Check sheet for the modelled part. Datum: model origin and axes. Units: mm. A direction names the side the tool comes from. Give positions to 0.01 mm unless a question says otherwise; leave off trailing zeros. Loops run counter-clockwise (first coordinate to the right, second up) from the corner with the lowest first, then second, coordinate; pieces in that order, holes last. Notation, with made-up numbers: (49.5, 7.25) - (75.5, 7.25) arc R21 ccw to (75.5, 42.25) - close; hole circle Ø1 at (33.5, -17). An arc over 180 degrees is marked (long way). Answer in a Markdown table with one row per item. Add a question column.
(1) Sectioned sample at A-A on z = 4. Enter the section's corners in (x, y).
(2) Sectioned sample at C-C on x = -27. Enter the section's corners in (y, z).
(3) Sectioned sample at D-D on x = 16. Enter the section's corners in (y, z), then the cut area to 3 significant figures.
(4) Go/stop test with flat-tipped pins: P1, Ø1.5, axis at x = 17.5, y = -4.5, coming from the +Z side; P2, Ø1.2, axis at x = 3, z = 1.5, coming from the -Y side; P3, Ø1, axis at x = -4.5, z = 3.5, coming from the +Y side; P4, Ø1.2, axis at y = 1.5, z = 2, coming from the -X side. Record where each tip stops, or that it passes through.
(5) Sectioned sample at B-B on y = -13. Enter the section's corners in (x, z), then the cut area to 3 significant figures.
(6) Thickness scan on L1, parallel to Y at x = -27, z = 5.45; L2, parallel to Y at x = 27, z = 2.9; L3, parallel to Y at x = 0, z = 0.5. Record the ranges inside material, lowest first.
(7) Draft check along Y on faces 1 (the face through (0, 0, 0)), 2 (the face through (-29.43, 8.17, 1.23)), 3 (the face through (-21.43, -8.616, 1.232)), 4 (the face through (24.636, -11.234, 1.232)). Enter one of: released by +Y, released by -Y, zero draft, split by the parting line, or undercut.
(8) Set-up check for faces 5 (the face through (-25, 14, 4.8)), 6 (the face through (-22, 7.57, 1)), 7 (the face through (4, 14.05, 1)): record each of +Z, -Z, +X, -X, +Y, -Y from which the full face is reachable in a straight line by a thin tool's end or side.
from build123d import *

# Parameters (mm, degrees)
SKETCH003_R   = 1.6
PAD_DEPTH     = 2.5
SKETCH_R      = 3
SKETCH_R_2    = 1.6
PAD001_DEPTH  = 2.3
SKETCH004_R   = 3
SKETCH004_R_2 = 2.5
PAD002_DEPTH  = 2
SKETCH005_W   = 26.6
SKETCH005_H   = 19.6
POCKET_DEPTH  = 1.5


with BuildPart() as part:
    # Sketch003 → Pad (new body)
    with BuildSketch(Plane.XY):
        with BuildLine():
            ThreePointArc((-28.087018, -11.203861), (-29.796139, -15.087018), (-25.912982, -16.796139))
            Line((-25.912982, -16.796139), (-0.93534, -7.085908))
            ThreePointArc((-0.210661, -6.95), (-0.579317, -6.984271), (-0.93534, -7.085908))
            Line((9.827812, -6.95), (-0.210661, -6.95))
            ThreePointArc((11.802562, -8.6332), (11.125194, -7.427896), (9.827812, -6.95))
            ThreePointArc((11.802562, -8.6332), (15.79003, -15.309423), (23.276895, -17.411493))
            Line((23.276895, -17.411493), (27.316256, -16.983284))
            ThreePointArc((27.316256, -16.983284), (29.983284, -13.683744), (26.683744, -11.016716))
            Line((22.644383, -11.444926), (26.683744, -11.016716))
            ThreePointArc((17.67, -6.97), (19.160409, -10.315499), (22.644383, -11.444926))
            Line((17.67, 14.05), (17.67, -6.97))
            Line((17.67, 14.05), (-10.570113, 14.05))
            ThreePointArc((-10.570113, 14.05), (-11.282503, 13.751783), (-11.57, 13.035))
            ThreePointArc((-12.569887, 12.02), (-11.857497, 12.318217), (-11.57, 13.035))
            Line((-23, 12.02), (-12.569887, 12.02))
            ThreePointArc((-24, 13.02), (-23.707107, 12.312893), (-23, 12.02))
            Line((-24, 13.02), (-24, 14))
            ThreePointArc((-24, 14), (-27, 17), (-30, 14))
            Line((-30, 14), (-30, 9.57))
            ThreePointArc((-30, 9.57), (-29.414214, 8.155786), (-28, 7.57))
            Line((-17.12, 7.57), (-28, 7.57))
            ThreePointArc((-14.583624, -5.954324), (-10.239947, 1.860298), (-17.12, 7.57))
            Line((-28.087018, -11.203861), (-14.583624, -5.954324))
        make_face()
        with Locations((-27, 14)):
            Circle(SKETCH003_R, mode=Mode.SUBTRACT)
        with Locations((27, -14)):
            Circle(SKETCH003_R, mode=Mode.SUBTRACT)
        with Locations((-27, -14)):
            Circle(SKETCH003_R, mode=Mode.SUBTRACT)
    extrude(amount=PAD_DEPTH)

    # Sketch → Pad001 (new body)
    with BuildSketch(Plane.XY.offset(2.5)):
        with Locations((-27, 14)):
            Circle(SKETCH_R)
        with Locations((-27, 14)):
            Circle(SKETCH_R_2, mode=Mode.SUBTRACT)
        with Locations((27, -14)):
            Circle(SKETCH_R)
        with Locations((27, -14)):
            Circle(SKETCH_R_2, mode=Mode.SUBTRACT)
        with Locations((-27, -14)):
            Circle(SKETCH_R)
        with Locations((-27, -14)):
            Circle(SKETCH_R_2, mode=Mode.SUBTRACT)
    extrude(amount=PAD001_DEPTH)

    # Sketch004 → Pad002 (new body)
    with BuildSketch(Plane.XY.offset(4.8)):
        with Locations((-27, 14)):
            Circle(SKETCH004_R)
        with Locations((-27, 14)):
            Circle(SKETCH004_R_2, mode=Mode.SUBTRACT)
        with Locations((-27, -14)):
            Circle(SKETCH004_R)
        with Locations((-27, -14)):
            Circle(SKETCH004_R_2, mode=Mode.SUBTRACT)
        with Locations((27, -14)):
            Circle(SKETCH004_R)
        with Locations((27, -14)):
            Circle(SKETCH004_R_2, mode=Mode.SUBTRACT)
    extrude(amount=PAD002_DEPTH)

    # Sketch005 → Pocket (cut)
    with BuildSketch(Plane.XY.offset(2.5)):
        with Locations((3.67, 3.55)):
            Rectangle(SKETCH005_W, SKETCH005_H)
    extrude(amount=-POCKET_DEPTH, mode=Mode.SUBTRACT)


solid = part.part
Reply:
| question | item | result |
|---|---|---|
| 1 | outline | circle Ø6 at (-27, -14); circle Ø6 at (-27, 14); circle Ø6 at (27, -14); hole circle Ø3.2 at (-27, -14); hole circle Ø3.2 at (-27, 14); hole circle Ø3.2 at (27, -14) |
| 2 | outline | (-17, 0) - (-15.6, 0) - (-15.6, 4.8) - (-16.5, 4.8) - (-16.5, 6.8) - (-17, 6.8) - close; (-12.4, 0) - (-10.78, 0) - (-10.78, 2.5) - (-11, 2.5) - (-11, 6.8) - (-11.5, 6.8) - (-11.5, 4.8) - (-12.4, 4.8) - close; (7.57, 0) - (12.4, 0) - (12.4, 4.8) - (11.5, 4.8) - (11.5, 6.8) - (11, 6.8) - (11, 2.5) - (7.57, 2.5) - close; (15.6, 0) - (17, 0) - (17, 6.8) - (16.5, 6.8) - (16.5, 4.8) - (15.6, 4.8) - close |
| 3 | outline | (-15.47, 0) - (14.05, 0) - (14.05, 2.5) - (13.35, 2.5) - (13.35, 1) - (-6.25, 1) - (-6.25, 2.5) - (-15.47, 2.5) - close |
| 3 | area | 44.4 mm^2 |
| 4 | P1 | z = 2.5 |
| 4 | P2 | y = -6.95 |
| 4 | P3 | through |
| 4 | P4 | x = -10.29 |
| 5 | outline | (-29.83, 0) - (-28.25, 0) - (-28.25, 4.8) - (-29.29, 4.8) - (-29.29, 6.8) - (-29.83, 6.8) - close; (-25.75, 0) - (-16.15, 0) - (-16.15, 2.5) - (-24.17, 2.5) - (-24.17, 6.8) - (-24.71, 6.8) - (-24.71, 4.8) - (-25.75, 4.8) - close; (13.57, 0) - (25.75, 0) - (25.75, 4.8) - (24.71, 4.8) - (24.71, 6.8) - (24.17, 6.8) - (24.17, 2.5) - (13.57, 2.5) - close; (28.25, 0) - (29.83, 0) - (29.83, 6.8) - (29.29, 6.8) - (29.29, 4.8) - (28.25, 4.8) - close |
| 5 | area | 81.2 mm^2 |
| 6 | L1 | -17 to -16.5, -11.5 to -11, 11 to 11.5, 16.5 to 17 |
| 6 | L2 | -17 to -15.6, -12.4 to -11 |
| 6 | L3 | -6.95 to 14.05 |
| 7 | face 1 | zero draft |
| 7 | face 2 | undercut |
| 7 | face 3 | undercut |
| 7 | face 4 | released by +Y |
| 8 | face 5 | +Z |
| 8 | face 6 | +Z, -Z, -X |
| 8 | face 7 | +Z, -Z, +X, +Y |
